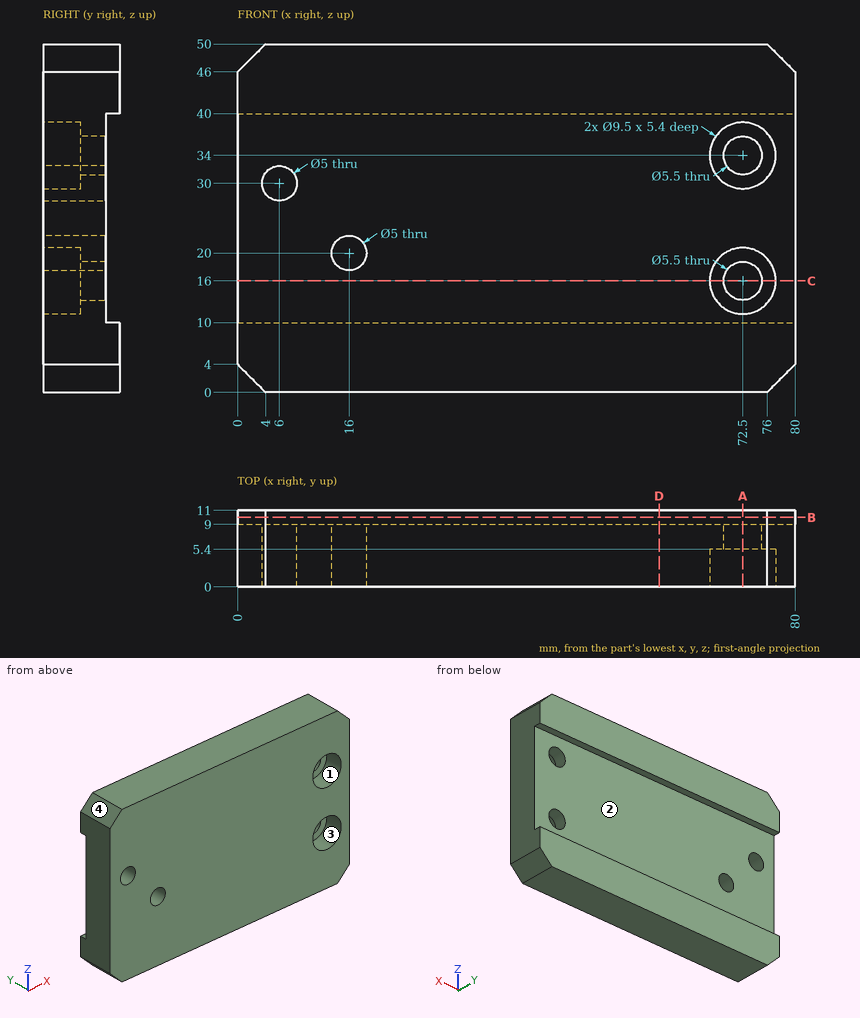
Source: three-view drawing plus pictorial views. Frame: mm from the lowest corner of the part. Give positions to 0.01 mm unless a question says otherwise; leave off trailing zeros. Loops run counter-clockwise (first coordinate to the right, second up) from the corner with the lowest first, then second, coordinate; pieces in that order, holes last. Notation, with made-up numbers: (53.5, 13) -> (61.5, 13) arc R29 cw to (61.5, 46) -> close; hole circle Ø10 at (33.25, -20). An arc over 180 degrees is marked (long way). Use a Markdown table: item, result. Add a question column.
(1) Section query B-B (y = 10). Output: boundary loops of the cut face in (x, z).
(2) First-contact query: pin 1 Ø10.5 at (x, z) = (72, 16.5) entering from -Y; pin 2 Ø7 at (x, z) = (72.5, 34) entering from +Y; pin 3 Ø8.5 at (x, z) = (72.5, 34) entering from -Y. Flat tips, straight axial feed; report the tip coordinate or a pass-through.
(3) Section query D-D (x = 60.5). Output: boundary loops of the cut face in (y, z), then the cut area to 3 significant figures.
(4) Section query A-A (x = 72.5). Output: boundary loops of the cut face in (y, z).
(5) Pull-direction query (X, two-part tool) for the marked faces 1, 2, 3 and 4; classes: +X half, -X half, draft (parallel to the pull), parting line (faces both ways), or undercut.
(6) Section query C-C (z = 16). Output: boundary loops of the cut face in (x, y), then the cut area to 3 significant figures.
(7) Ray query, line 1 (Z direction, x = 72.5, y = 6.95); line 2 (Z direction, x = 44, y = 10); line 3 (X direction, y = 7.25, z = 30). Return the intervals inside material, ascending.
Checked values:
| question | item | result |
|---|---|---|
| 1 | outline | (0, 4) -> (4, 0) -> (76, 0) -> (80, 4) -> (80, 10) -> (0, 10) -> close; (0, 40) -> (80, 40) -> (80, 46) -> (76, 50) -> (4, 50) -> (0, 46) -> close |
| 2 | pin 1 | y = 0 |
| 2 | pin 2 | y = 9 |
| 2 | pin 3 | y = 5.4 |
| 3 | outline | (0, 0) -> (11, 0) -> (11, 10) -> (9, 10) -> (9, 40) -> (11, 40) -> (11, 50) -> (0, 50) -> close |
| 3 | area | 490 mm^2 |
| 4 | outline | (0, 0) -> (11, 0) -> (11, 10) -> (9, 10) -> (9, 13.25) -> (5.4, 13.25) -> (5.4, 11.25) -> (0, 11.25) -> close; (0, 20.75) -> (5.4, 20.75) -> (5.4, 18.75) -> (9, 18.75) -> (9, 31.25) -> (5.4, 31.25) -> (5.4, 29.25) -> (0, 29.25) -> close; (0, 38.75) -> (5.4, 38.75) -> (5.4, 36.75) -> (9, 36.75) -> (9, 40) -> (11, 40) -> (11, 50) -> (0, 50) -> close |
| 5 | face 1 | undercut |
| 5 | face 2 | draft |
| 5 | face 3 | undercut |
| 5 | face 4 | -X half |
| 6 | outline | (0, 0) -> (67.75, 0) -> (67.75, 5.4) -> (69.75, 5.4) -> (69.75, 9) -> (0, 9) -> close; (75.25, 5.4) -> (77.25, 5.4) -> (77.25, 0) -> (80, 0) -> (80, 9) -> (75.25, 9) -> close |
| 6 | area | 649 mm^2 |
| 7 | line 1 | 0 to 13.25, 18.75 to 31.25, 36.75 to 50 |
| 7 | line 2 | 0 to 10, 40 to 50 |
| 7 | line 3 | 0 to 3.5, 8.5 to 80 |
